Part model, mm, in its own coordinate system. Give positions to 0.01 mm unless a question says otherwise; leave off trailing zeros. Write each loop counter-clockwise with the first axis right and the second up, starting at its lowest first coordinate (ties: lowest second). Pieces come first, ordered by that corner, then holes.
```python
from build123d import *

# Parameters (mm, degrees)
F0_W     = 203.2
F0_H     = 101.6
F1_DEPTH = 19.05
F2_SIZE2 = 2.339036
F2_SIZE  = 19.04999
F3_SIZE2 = 2.339036
F3_SIZE  = 19.04999


# Not quite as in the source:
# - a fillet or chamfer is up to 0.001 mm smaller than in the source, because OpenCascade refuses the exact size


with BuildPart() as f1:
    # F0 (on Front) → F1 (new body)
    with BuildSketch(Plane.XZ):
        Rectangle(F0_W, F0_H)
    extrude(amount=F1_DEPTH)

    # F2 (size 19.05 and 2.3390458852 in the source; OpenCascade refuses exactly that, so slightly less here)
    f2_edges = [f1.edges().sort_by_distance(p)[0] for p in [
        (-101.6, 0, 0),
    ]]
    f2_side = f1.faces().sort_by_distance((-101.6, -9.525, 0))[0]
    chamfer(f2_edges, length=F2_SIZE, length2=F2_SIZE2, reference=f2_side)

    # F3 (size 19.05 and 2.3390458852 in the source; OpenCascade refuses exactly that, so slightly less here)
    f3_edges = [f1.edges().sort_by_distance(p)[0] for p in [
        (101.6, 0, 0),
    ]]
    f3_side = f1.faces().sort_by_distance((101.6, -9.525, 0))[0]
    chamfer(f3_edges, length=F3_SIZE, length2=F3_SIZE2, reference=f3_side)


solid = f1.part
```
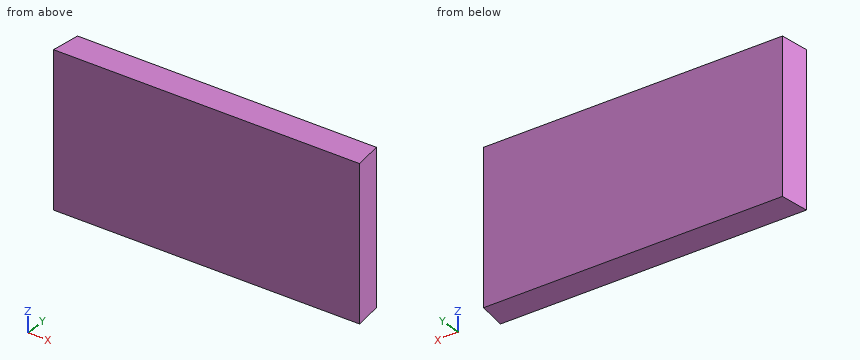
1) Wall check: L1, parallel to X at y = -11, z = 2; L2, parallel to X at y = -2.75, z = -13.5. Give the ranges that are in metal, low to high.
Answers follow:
L1: x = -100.61 to 100.61
L2: x = -99.6 to 99.6
2) Pin check, flat tips, straight feed: pin 1 Ø1.5 at (x, z) = (47.5, 29.5) entering from +Y; pin 2 Ø1 at (y, z) = (-2.5, -27) entering from +X; pin 3 Ø3 at (y, z) = (-5, -36.5) entering from -X; pin 4 Ø1.5 at (y, z) = (-10, 18.5) entering from +X. Stop position of each tip, or through.
Answers follow:
pin 1: stops at y = 0
pin 2: stops at x = 99.63
pin 3: stops at x = -100.06
pin 4: stops at x = 100.58
3) Saw through at A-A, the plane y = -4.25. Write the cut outline in (x, z).
Answers follow:
outline: (-99.78, -50.8) - (99.78, -50.8) - (99.78, 50.8) - (-99.78, 50.8) - close
